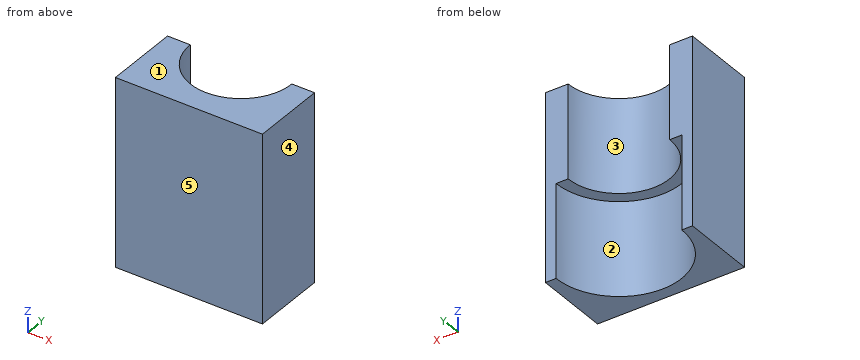
```python
from build123d import *

# Parameters (mm, degrees)
BOSS_EXTRUDE1_DEPTH = 35
BOSS_EXTRUDE2_DEPTH = 35


with BuildPart() as part:
    # Sketch2 → Boss-Extrude1 (new body)
    with BuildSketch(Plane.XY):
        with BuildLine():
            Line((48.748941829, 15.932254861), (44.748941829, 15.932254861))
            Line((44.748941829, 15.932254861), (44.748941829, -12.067745139))
            Line((44.748941829, -12.067745139), (99.748941829, -12.067745139))
            Line((99.748941829, -12.067745139), (99.748941829, 15.932254861))
            Line((99.748941829, 15.932254861), (95.748941829, 15.932254861))
            ThreePointArc((95.748941829, 15.932254861), (72.248941829, -7.567745139), (48.748941829, 15.932254861))
        make_face()
    extrude(amount=BOSS_EXTRUDE1_DEPTH)

    # Sketch3 → Boss-Extrude2 (add)
    with BuildSketch(Plane.XY.offset(35)):
        with BuildLine():
            Line((91.248941829, 15.932254861), (99.748941829, 15.932254861))
            Line((99.748941829, 15.932254861), (99.748941829, -12.067745139))
            Line((99.748941829, -12.067745139), (44.748941829, -12.067745139))
            Line((44.748941829, -12.067745139), (44.748941829, 15.932254861))
            Line((44.748941829, 15.932254861), (53.248941829, 15.932254861))
            ThreePointArc((53.248941829, 15.932254861), (72.248941829, -3.067745139), (91.248941829, 15.932254861))
        make_face()
    extrude(amount=BOSS_EXTRUDE2_DEPTH)


solid = part.part
```
For this review, take the finished solid that the model builds, in its own axes (mm). Face numbers are marked on the shaded views. A direction names the side the tool comes from. Give positions to 0.01 mm unless a question says otherwise; leave off trailing zeros. Loops run counter-clockwise (first coordinate to the right, second up) from the corner with the lowest first, then second, coordinate; pieces in that order, holes last. Notation, with made-up numbers: M 70,58 L 119,58 A12 cw 119,69 Z; hole C 33.25,53.25 d7. An arc over 180 degrees is marked long. One line per item, written item: value. Start each with the question number.
Q1. For L1, parallel to X at y = 4, z = 54; L2, parallel to X at y = 3, z = 22; L3, parallel to Z at x = 91, y = 7.25, list the stretches that pass through material, from the lowest coordinate up.
Q2. Add section B-B (z = 49). Give the boundary of the cut face in (x, y), and give its area (3 significant figures).
Q3. Add section A-A (y = 12.5). Give the boundary of the cut face in (x, z).
Q4. Draft analysis for pull direction X (two halves, no side actions). For the marked faces 3, 4 and 5, state which applies: released by +X, released by -X, zero draft, split by the parting line, or undercut.
Q5. Add section D-D (y = 5). Give the boundary of the cut face in (x, z), and give its area (3 significant figures).
Q6. Machinability: for the marked faces 1 and 2, which of the approach directions +Z, -Z, +X, -X, +Y, -Y give a long, thin tool a straight path to every point of the face, cutting with its end or side? Answer none if there is none.
Q7. Clearance check with flat-ended pins moving along their axes: pin 1 Ø8 at (x, y) = (61, 1) entering from +Z; pin 2 Ø4 at (x, z) = (60, 51) entering from +Y; pin 3 Ø10 at (x, z) = (78.5, 49) entering from +Y. State where each tip first meets the part, or that it passes through.
Q8. Add section C-C (x = 84.5). Give the boundary of the cut face in (y, z), and give its area (3 significant figures).
Reply:
1. L1: 44.75 to 57.46, 87.03 to 99.75
1. L2: 44.75 to 52.63, 91.87 to 99.75
1. L3: 35 to 70
2. outline: M 44.75,-12.07 L 99.75,-12.07 L 99.75,15.93 L 91.25,15.93 A19 cw 53.25,15.93 L 44.75,15.93 Z
2. area: 973 mm²
3. outline: M 44.75,0 L 49,0 L 49,35 L 53.56,35 L 53.56,70 L 44.75,70 Z; M 90.94,35 L 95.5,35 L 95.5,0 L 99.75,0 L 99.75,70 L 90.94,70 Z
4. face 3: undercut
4. face 4: released by +X
4. face 5: zero draft
5. outline: M 44.75,0 L 51.45,0 L 51.45,35 L 56.71,35 L 56.71,70 L 44.75,70 Z; M 87.79,35 L 93.05,35 L 93.05,0 L 99.75,0 L 99.75,70 L 87.79,70 Z
5. area: 1,310 mm²
6. face 1: +Z, +X, -X, +Y, -Y
6. face 2: -Z, +Y
7. pin 1: z = 70
7. pin 2: y = 3.36
7. pin 3: y = 0.62
8. outline: M -12.07,0 L -4.12,0 L -4.12,35 L 1.41,35 L 1.41,70 L -12.07,70 Z
8. area: 750 mm²
